from build123d import *

# Parameters (mm, degrees)
EXTRUDE_1_DEPTH     = 17
CUT_EXTRUDE_1_DEPTH = 15
CUT_EXTRUDE_2_DEPTH = 15
CUT_EXTRUDE_3_DEPTH = 15
CUT_EXTRUDE_4_DEPTH = 15
CUT_EXTRUDE_5_DEPTH = 15
CUT_EXTRUDE_6_DEPTH = 15
CUT_EXTRUDE_7_DEPTH = 18
FILLET_1_R          = 2
FILLET_2_R          = 3


with BuildPart() as part:
    # 草图1 → 凸台-拉伸1 (new body)
    with BuildSketch(Plane(origin=(0, 0, 0), x_dir=(-1, 0, 0), z_dir=(0, 0, -1))):
        with BuildLine():
            Line((-10.093009514, -187.6), (-89.906992274, -187.6))
            ThreePointArc((-89.906992274, -187.6), (-91.240663452, -187.689332959), (-92.550506472, -187.955735762))
            ThreePointArc((-92.550506472, -187.955735762), (-50.000000894, -247.6), (-7.449495316, -187.955735762))
            ThreePointArc((-7.449495316, -187.955735762), (-8.759338336, -187.689332959), (-10.093009514, -187.6))
        make_face()
    extrude(amount=-EXTRUDE_1_DEPTH)

    # 草图2 → 切除-拉伸1 (cut)
    with BuildSketch(Plane.XY.offset(17)):
        with BuildLine():
            ThreePointArc((6.138583991, -212.658633467), (6.427726824, -211.707087742), (7.394913242, -211.47558552))
            ThreePointArc((7.394913242, -211.47558552), (19.250000894, -202.6), (7.394913242, -193.72441448))
            ThreePointArc((7.394913242, -193.72441448), (6.427726824, -193.492912258), (6.138583991, -192.541366533))
            ThreePointArc((6.138583991, -192.541366533), (5.000000894, -202.6), (6.138583991, -212.658633467))
        make_face()
    extrude(amount=-CUT_EXTRUDE_1_DEPTH, mode=Mode.SUBTRACT)

    # 草图3 → 切除-拉伸2 (cut)
    with BuildSketch(Plane.XY.offset(17)):
        with BuildLine():
            ThreePointArc((20.558692873, -236.632475402), (20.195546949, -235.606932185), (20.891610548, -234.770804613))
            ThreePointArc((20.891610548, -234.770804613), (25.122728317, -220.674396508), (10.408760237, -220.342398969))
            ThreePointArc((10.408760237, -220.342398969), (9.398460179, -220.746017161), (8.535328882, -220.083734582))
            ThreePointArc((8.535328882, -220.083734582), (13.594236147, -229.050336353), (20.558692873, -236.632475402))
        make_face()
    extrude(amount=-CUT_EXTRUDE_2_DEPTH, mode=Mode.SUBTRACT)

    # 草图4 → 切除-拉伸3 (cut)
    with BuildSketch(Plane.XY.offset(17)):
        with BuildLine():
            ThreePointArc((46.35614853, -247.452227815), (45.378748434, -246.7903036), (45.441184322, -245.611509143))
            ThreePointArc((45.441184322, -245.611509143), (40.497728317, -231.844987876), (28.406630222, -240.076646999))
            ThreePointArc((28.406630222, -240.076646999), (27.764263919, -241.067010643), (26.584461339, -241.028017219))
            ThreePointArc((26.584461339, -241.028017219), (36.094236147, -245.397543233), (46.35614853, -247.452227815))
        make_face()
    extrude(amount=-CUT_EXTRUDE_3_DEPTH, mode=Mode.SUBTRACT)

    # 草图5 → 切除-拉伸4 (cut)
    with BuildSketch(Plane.XY.offset(17)):
        with BuildLine():
            ThreePointArc((73.560141987, -240.939532492), (72.289088744, -240.990132521), (71.583355923, -239.931795197))
            ThreePointArc((71.583355923, -239.931795197), (59.502273471, -231.844987876), (54.481778538, -245.488434526))
            ThreePointArc((54.481778538, -245.488434526), (54.532903764, -246.759466752), (53.474858139, -247.465636818))
            ThreePointArc((53.474858139, -247.465636818), (63.905765641, -245.397543233), (73.560141987, -240.939532492))
        make_face()
    extrude(amount=-CUT_EXTRUDE_4_DEPTH, mode=Mode.SUBTRACT)

    # 草图6 → 切除-拉伸5 (cut)
    with BuildSketch(Plane.XY.offset(17)):
        with BuildLine():
            ThreePointArc((91.659654246, -219.613914382), (90.59547429, -220.46525304), (89.311552324, -220.008305698))
            ThreePointArc((89.311552324, -220.008305698), (74.877273471, -220.674396508), (78.704220933, -234.608044849))
            ThreePointArc((78.704220933, -234.608044849), (79.535557387, -235.687922708), (79.0547359, -236.963096102))
            ThreePointArc((79.0547359, -236.963096102), (86.405765641, -229.050336353), (91.659654246, -219.613914382))
        make_face()
    extrude(amount=-CUT_EXTRUDE_5_DEPTH, mode=Mode.SUBTRACT)

    # 草图7 → 切除-拉伸6 (cut)
    with BuildSketch(Plane.XY.offset(17)):
        with BuildLine():
            ThreePointArc((93.664063394, -191.716542553), (93.288877928, -193.119991574), (91.900418772, -193.547325705))
            ThreePointArc((91.900418772, -193.547325705), (80.750000894, -202.6), (91.900418772, -211.652674295))
            ThreePointArc((91.900418772, -211.652674295), (93.288877928, -212.080008426), (93.664063394, -213.483457447))
            ThreePointArc((93.664063394, -213.483457447), (95.000000894, -202.6), (93.664063394, -191.716542553))
        make_face()
    extrude(amount=-CUT_EXTRUDE_6_DEPTH, mode=Mode.SUBTRACT)

    # 草图8 → 切除-拉伸7 (cut, through all)
    with BuildSketch(Plane.XY.offset(17)):
        with BuildLine():
            Line((77.500000894, -187.6), (22.500000894, -187.6))
            Line((22.500000894, -187.6), (22.500000894, -202.6))
            ThreePointArc((22.500000894, -202.6), (50.000000894, -230.1), (77.500000894, -202.6))
            Line((77.500000894, -202.6), (77.500000894, -187.6))
        make_face()
    extrude(amount=-CUT_EXTRUDE_7_DEPTH, mode=Mode.SUBTRACT)

    # 圆角1
    fillet_1_edges = [part.edges().sort_by_distance(p)[0] for p in [
        (92.550506472, -187.955735762, 8.5),
        (7.449495316, -187.955735762, 8.5),
    ]]
    fillet(fillet_1_edges, radius=FILLET_1_R)

    # 圆角2
    fillet_2_edges = [part.edges().sort_by_distance(p)[0] for p in [
        (77.500000894, -187.6, 8.5),
        (22.500000894, -187.6, 8.5),
    ]]
    fillet(fillet_2_edges, radius=FILLET_2_R)


solid = part.part
For this review, take the finished solid that the model builds, in its own axes (mm). A direction names the side the tool comes from. Give positions to 0.01 mm unless a question says otherwise; leave off trailing zeros. Order: outer loops, then holes, each group sorted by start corner. A loop starts at its lowest first (then second) coordinate and runs counter-clockwise, first axis right, second up. Notation, with made-up numbers: M 12.5,87.5 L 42.5,87.5 A16 cw 42.5,95.5 Z; hole C -30.5,-0.5 d9. An arc over 180 degrees is marked long. Answer in a Markdown table with one row per item. Add a question column.
(1) For pin 1 (2 mm diameter, centred on x = 30, y = -238.5, fed in from +Z); pin 2 (4 mm diameter, centred on x = 59.5, z = 10.5, fed in from +Y); pin 3 (4 mm diameter, centred on y = -196.5, z = 9.5, fed in from +X), all flat-tipped, find the tip position at first contact; note any pin that passes through.
(2) Consider section A-A on y = -201.5. State the section outline as (x, z) points, and give its area (3 significant figures).
(3) Consider section B-B on x = 84. State the section outline as (y, z) points, and give its area (3 significant figures).
(4) Consider section D-D on x = 24.5. State the section outline as (y, z) points, and give its area (3 significant figures).
(5) Consider section C-C on y = -233.5. State the section outline as (x, z) points.
(6) Mouldability with a two-part tool opening along X and no side actions: class faces 4 (the face through (75.016, -220.488, 9.605)), 5 (the face through (51.182, -247.584, 6.492)), 6 (the face through (54.541, -246.743, 9.605)), 7 (the face through (50, -231, 17)) as +X half, -X half, draft (parallel to the pull), parting line (faces both ways), or undercut.
(7) For faces 1 (the face through (21.6, -188.46, 8.38)), 2 (the face through (59.726, -231.775, 9.605)), 3 (the face through (90.62, -220.46, 9.6)), list the 3-axis set-ups (+Z, -Z, +X, -X, +Y, -Y) from which the entire face can be reached by the end or side of a thin tool; tool diameter is ignored.
(8) Wall thickness on probe 1 along X at (y, z) = (-240.5, 3.75); probe 2 along X at (y, z) = (-202.6, 8.5); probe 3 along X at (y, z) = (-241, 8.5): over which ranges is each line inside the solid? List them lowest first. Write a range as [from, to].
Evaluation:
| question | item | result |
|---|---|---|
| 1 | pin 1 | stops at z = 2 |
| 1 | pin 2 | stops at y = -227.58 |
| 1 | pin 3 | stops at x = 85.53 |
| 2 | outline | M 5.01,0 L 22.5,0 L 22.5,17 L 19.18,17 L 19.18,2 L 5.01,2 Z; M 77.5,0 L 94.99,0 L 94.99,2 L 80.82,2 L 80.82,17 L 77.5,17 Z |
| 2 | area | 169 mm^2 |
| 3 | outline | M -232.08,0 L -187.6,0 L -187.6,17 L -195.56,17 L -195.56,2 L -209.64,2 L -209.64,17 L -217.01,17 L -217.01,2 L -232.08,2 Z |
| 3 | area | 319 mm^2 |
| 4 | outline | M -239.68,0 L -212.9,0 L -212.9,17 L -219.91,17 L -219.91,2 L -232.32,2 L -232.32,17 L -239.68,17 Z |
| 4 | area | 269 mm^2 |
| 5 | outline | M 17.29,0 L 82.71,0 L 82.71,2 L 76.8,2 L 76.8,17 L 68.24,17 L 68.24,2 L 56.48,2 L 56.48,17 L 43.52,17 L 43.52,2 L 31.76,2 L 31.76,17 L 23.2,17 L 23.2,2 L 17.29,2 Z |
| 6 | face 4 | undercut |
| 6 | face 5 | parting line |
| 6 | face 6 | +X half |
| 6 | face 7 | draft |
| 7 | face 1 | +Z, -Z, +Y |
| 7 | face 2 | +Z |
| 7 | face 3 | +Z, -Y |
| 8 | probe 1 | x = [25.74, 28.3], [46.89, 53.11], [71.76, 74.26] |
| 8 | probe 2 | x = [19.25, 22.5], [77.5, 80.75] |
| 8 | probe 3 | x = [26.54, 27.88], [46.88, 53.12], [72.31, 73.45] |
